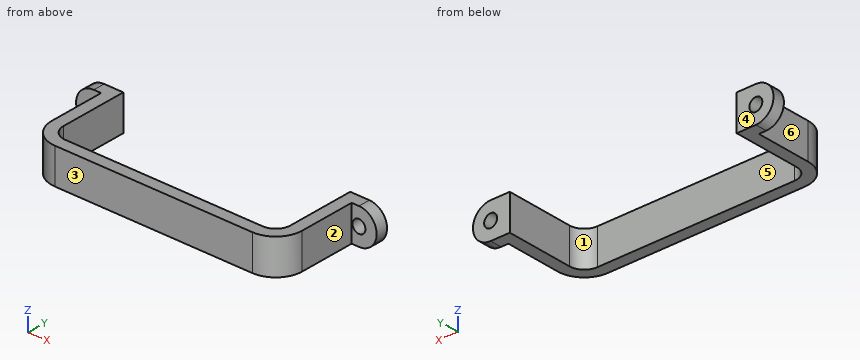
```python
from build123d import *

# Parameters (mm, degrees)
BOSS_EXTRUDE1_DEPTH = 6
SKETCH3_R           = 1.1
BOSS_EXTRUDE6_DEPTH = 2


with BuildPart() as part:
    # Sketch1 → Boss-Extrude1 (new body)
    with BuildSketch(Plane.XY):
        with BuildLine():
            Line((-21.25, 14), (-21.25, 2.5))
            ThreePointArc((-21.25, 2.5), (-19.931980515, -0.681980515), (-16.75, -2))
            Line((-16.75, -2), (16.75, -2))
            ThreePointArc((16.75, -2), (19.931980515, -0.681980515), (21.25, 2.5))
            Line((21.25, 2.5), (21.25, 14))
            Line((21.25, 14), (19.25, 14))
            Line((19.25, 14), (19.25, 2.5))
            ThreePointArc((19.25, 2.5), (18.517766953, 0.732233047), (16.75, 0))
            Line((16.75, 0), (-16.75, 0))
            ThreePointArc((-16.75, 0), (-18.517766953, 0.732233047), (-19.25, 2.5))
            Line((-19.25, 2.5), (-19.25, 14))
            Line((-19.25, 14), (-21.25, 14))
        make_face()
    extrude(amount=BOSS_EXTRUDE1_DEPTH)

    # Sketch3 → Boss-Extrude6 (add)
    # profile 1 of 2: a face of its own
    with BuildSketch(Plane(origin=(0, 14, 0), x_dir=(-1, 0, 0), z_dir=(0, 1, 0))):
        with BuildLine():
            Line((-21.25, 6), (-22.5, 6))
            ThreePointArc((-22.5, 6), (-25.5, 3), (-22.5, 0))
            Line((-22.5, 0), (-21.25, 0))
            Line((-21.25, 0), (-21.25, 6))
        make_face()
        with Locations(Location((-22.5, 3, 0), (0, 0, 90))):
            Circle(SKETCH3_R, mode=Mode.SUBTRACT)
    # profile 2 of 2: a face of its own
    with BuildSketch(Plane(origin=(0, 14, 0), x_dir=(-1, 0, 0), z_dir=(0, 1, 0))):
        with BuildLine():
            Line((22.5, 6), (21.25, 6))
            Line((21.25, 6), (21.25, 0))
            Line((21.25, 0), (22.5, 0))
            ThreePointArc((22.5, 0), (25.5, 3), (22.5, 6))
        make_face()
        with Locations(Location((22.5, 3, 0), (0, 0, 90))):
            Circle(SKETCH3_R, mode=Mode.SUBTRACT)
    extrude(amount=-BOSS_EXTRUDE6_DEPTH)


solid = part.part
```
The model under review builds one solid part; all positions refer to its coordinate system, in mm. Face numbers are marked on the shaded views. A direction names the side the tool comes from. Give positions to 0.01 mm unless a question says otherwise; leave off trailing zeros. Write each loop counter-clockwise with the first axis right and the second up, starting at its lowest first coordinate (ties: lowest second). Pieces come first, ordered by that corner, then holes. Notation, with made-up numbers: M 28.5,15.25 L 71.5,15.25 A32 cw 71.5,47.25 Z; hole C -17.5,-2 d8. An arc over 180 degrees is marked long. Answer in a Markdown table with one row per item.
Item 1: Draft analysis for pull direction X (two halves, no side actions). For the marked faces 4, 5 and 6, state which applies: +X half, -X half, draft (parallel to the pull), parting line (faces both ways), or undercut.
Check sheet entries:
| item | result |
|---|---|
| face 4 | draft |
| face 5 | undercut |
| face 6 | -X half |
Item 2: Add section B-B on z = 3. Give the boundary of the cut face in (x, y), plus the area to 3 significant figures.
Check sheet entries:
| item | result |
|---|---|
| outline | M -25.5,12 L -23.6,12 L -23.6,14 L -25.5,14 Z; M -21.4,12 L -21.25,12 L -21.25,2.5 A4.5 ccw -16.75,-2 L 16.75,-2 A4.5 ccw 21.25,2.5 L 21.25,12 L 21.4,12 L 21.4,14 L 19.25,14 L 19.25,2.5 A2.5 cw 16.75,0 L -16.75,0 A2.5 cw -19.25,2.5 L -19.25,14 L -21.4,14 Z; M 23.6,12 L 25.5,12 L 25.5,14 L 23.6,14 Z |
| area | 143 mm2 |
Item 3: Add section C-C on y = 0.75. Give the boundary of the cut face in (x, z), plus the area to 3 significant figures.
Check sheet entries:
| item | result |
|---|---|
| outline | M -20.9,0 L -18.54,0 L -18.54,6 L -20.9,6 Z; M 18.54,0 L 20.9,0 L 20.9,6 L 18.54,6 Z |
| area | 28.3 mm2 |
Item 4: For line 1 along X through (y, z) = (13.55, 3); line 2 along X through (y, z) = (3, 4.25); line 3 along Y through (x, z) = (0, 2.85), list the stretches that pass through material, from the lowest coordinate up.
Check sheet entries:
| item | result |
|---|---|
| line 1 | -25.5 to -23.6, -21.4 to -19.25, 19.25 to 21.4, 23.6 to 25.5 |
| line 2 | -21.25 to -19.25, 19.25 to 21.25 |
| line 3 | -2 to 0 |
Item 5: Add section A-A on y = 4.25. Give the boundary of the cut face in (x, z).
Check sheet entries:
| item | result |
|---|---|
| outline | M -21.25,0 L -19.25,0 L -19.25,6 L -21.25,6 Z; M 19.25,0 L 21.25,0 L 21.25,6 L 19.25,6 Z |
Item 6: For P1, Ø3, axis at y = 7.5, z = 1.5, coming from the +X side; P2, Ø3, axis at y = 6.5, z = 2, coming from the -X side; P3, Ø3, axis at x = 1, z = 4, coming from the +Y side, all flat-tipped, find the tip position at first contact; note any pin that passes through.
Check sheet entries:
| item | result |
|---|---|
| P1 | x = 21.25 |
| P2 | x = -21.25 |
| P3 | y = 0 |
Item 7: Add section D-D on z = 5.05. Give the boundary of the cut face in (x, y).
Check sheet entries:
| item | result |
|---|---|
| outline | M -24.69,12 L -21.25,12 L -21.25,2.5 A4.5 ccw -16.75,-2 L 16.75,-2 A4.5 ccw 21.25,2.5 L 21.25,12 L 24.69,12 L 24.69,14 L 19.25,14 L 19.25,2.5 A2.5 cw 16.75,0 L -16.75,0 A2.5 cw -19.25,2.5 L -19.25,14 L -24.69,14 Z |
Item 8: Tool access review of the marked faces 1, 2 and 3: name each direction out of +Z, -Z, +X, -X, +Y, -Y from which nothing blocks a thin tool from reaching the whole face with its end or side.
Check sheet entries:
| item | result |
|---|---|
| face 1 | +Z, -Z, +Y |
| face 2 | +Z, -Z, +X, -Y |
| face 3 | +Z, -Z, +X, -X, -Y |
